Can you work these out from the model? Positions are in its coordinate system, mm. A direction names the side the tool comes from. Give positions to 0.01 mm unless a question says otherwise; leave off trailing zeros. Write each loop counter-clockwise with the first axis right and the second up, starting at its lowest first coordinate (ties: lowest second). Pieces come first, ordered by that corner, then holes. Notation, with made-up numbers: (49, 0.25) -> (90, 0.25) arc R23 ccw to (90, 37.25) -> close; hole circle Ø6 at (59, -33). An arc over 180 degrees is marked (long way). One line per item, written item: value.
from build123d import *

# Parameters (mm, degrees)
SKETCH1_W           = 40
SKETCH1_H           = 20
SKETCH1_R           = 4
BOSS_EXTRUDE1_DEPTH = 38
SKETCH1_3_R         = 4
BOSS_EXTRUDE2_DEPTH = 6
SKETCH2_R           = 6.5
BOSS_EXTRUDE3_DEPTH = 2
SKETCH3_W           = 7
SKETCH3_H           = 20
SKETCH3_R           = 2.25
BOSS_EXTRUDE4_DEPTH = 2.5


with BuildPart() as part:
    # Sketch1 → Boss-Extrude1 (new body)
    # profile 1 of 2: a face of its own
    with BuildSketch(Plane(origin=(0, 0, 0), x_dir=(1, 0, 0), z_dir=(0, 1, 0))):
        with Locations((-11, 0)):
            Rectangle(SKETCH1_W, SKETCH1_H)
        Circle(SKETCH1_R, mode=Mode.SUBTRACT)
    # profile 2 of 2: a face of its own
    with BuildSketch(Plane(origin=(0, 0, 0), x_dir=(1, 0, 0), z_dir=(0, 1, 0))):
        Circle(SKETCH1_R)
    extrude(amount=-BOSS_EXTRUDE1_DEPTH)

    # Sketch1_3 → Boss-Extrude2 (add)
    with BuildSketch(Plane(origin=(0, 0, 0), x_dir=(1, 0, 0), z_dir=(0, 1, 0))):
        with Locations(Location((0, 0, 0), (0, 0, 270))):
            Circle(SKETCH1_3_R)
    extrude(amount=BOSS_EXTRUDE2_DEPTH)

    # Sketch2 → Boss-Extrude3 (add)
    with BuildSketch(Plane(origin=(0, 0, 0), x_dir=(1, 0, 0), z_dir=(0, 1, 0))):
        with Locations(Location((0, 0, 0), (0, 0, 270))):
            Circle(SKETCH2_R)
    extrude(amount=BOSS_EXTRUDE3_DEPTH)


with BuildPart() as body_2:
    # Sketch3 → Boss-Extrude4 (new body)
    with BuildSketch(Plane(origin=(0, -8, 0), x_dir=(-1, 0, 0), z_dir=(0, -1, 0))):
        with Locations((-12.5, 0)):
            Rectangle(SKETCH3_W, SKETCH3_H)
        with Locations(Location((-13.5, 5, 0), (0, 0, 90))):
            Circle(SKETCH3_R, mode=Mode.SUBTRACT)
        with Locations(Location((-13.5, -5, 0), (0, 0, 90))):
            Circle(SKETCH3_R, mode=Mode.SUBTRACT)
    extrude(amount=BOSS_EXTRUDE4_DEPTH)


with BuildPart() as body_3:
    # Mirror1: mirrored copy
    add(body_2.part.mirror(Plane(origin=(-11, 0, 0), x_dir=(0, 0, 1), z_dir=(1, 0, 0))))

    # Combine1: union part, body 2
    add(part.part)
    add(body_2.part)


solid = body_3.part
1) For faces 1 (the face through (-35, -10.5, 0)), 2 (the face through (3, 2, 3)), 3 (the face through (-31, -4, 0)), 4 (the face through (9, -24, 0)), 5 (the face through (13, -8, 0)), which set-ups out of +Z, -Z, +X, -X, +Y, -Y let a thin tool reach every point of the face, with its end or its side?
Answer list:
face 1: +Z, -Z, -X, -Y
face 2: +Y
face 3: +Z, -Z, -X, +Y
face 4: +Z, -Z, +X, -Y
face 5: +Z, -Z, +X, +Y
2) If we section it at C-C (x = 0): Write out the boundary of the cut face in (y, z), and give its area (3 significant figures).
Answer list:
outline: (-38, -10) -> (0, -10) -> (0, -6.5) -> (2, -6.5) -> (2, -4) -> (6, -4) -> (6, 4) -> (2, 4) -> (2, 6.5) -> (0, 6.5) -> (0, 10) -> (-38, 10) -> close
area: 818 mm^2
3) I need wall thicknesses on L1, parallel to X at y = -8.95, z = -5; L2, parallel to Z at x = -35.5, y = -9.3; L3, parallel to Y at x = 5, z = -4.75. Which ranges of each line are inside material? Lowest first, please.
Answer list:
L1: x = -38 to -37.75, -33.25 to 11.25, 15.75 to 16
L2: z = -10 to -7.25, -2.75 to 2.75, 7.25 to 10
L3: y = -38 to 0
4) Will these pins go through, and if not, where does the flat tip stop? pin 1 (5.5 mm diameter, centred on x = 12.5, z = -4.5, fed in from -Y); pin 2 (2 mm diameter, centred on y = -13.5, z = 3.5, fed in from +X); pin 3 (10 mm diameter, centred on y = -31.5, z = 5, fed in from -X); pin 4 (6 mm diameter, centred on x = -1, z = -5, fed in from +Y).
Answer list:
pin 1: stops at y = -10.5
pin 2: stops at x = 9
pin 3: stops at x = -31
pin 4: stops at y = 6
5) If we section it at A-A (x = 13.5): Write out the boundary of the cut face in (y, z).
Answer list:
outline: (-10.5, -10) -> (-8, -10) -> (-8, -7.25) -> (-10.5, -7.25) -> close; (-10.5, -2.75) -> (-8, -2.75) -> (-8, 2.75) -> (-10.5, 2.75) -> close; (-10.5, 7.25) -> (-8, 7.25) -> (-8, 10) -> (-10.5, 10) -> close
6) If we section it at B-B (z = 5): Write out the boundary of the cut face in (x, y), and give its area (3 significant figures).
Answer list:
outline: (-38, -10.5) -> (-37.75, -10.5) -> (-37.75, -8) -> (-38, -8) -> close; (-33.25, -10.5) -> (-31, -10.5) -> (-31, -38) -> (9, -38) -> (9, -10.5) -> (11.25, -10.5) -> (11.25, -8) -> (9, -8) -> (9, 0) -> (4.15, 0) -> (4.15, 2) -> (-4.15, 2) -> (-4.15, 0) -> (-31, 0) -> (-31, -8) -> (-33.25, -8) -> close; (15.75, -10.5) -> (16, -10.5) -> (16, -8) -> (15.75, -8) -> close
area: 1,550 mm^2
7) If we section it at D-D (z = 0): Write out the boundary of the cut face in (x, y), and give its area (3 significant figures).
Answer list:
outline: (-38, -10.5) -> (-31, -10.5) -> (-31, -38) -> (9, -38) -> (9, -10.5) -> (16, -10.5) -> (16, -8) -> (9, -8) -> (9, 0) -> (6.5, 0) -> (6.5, 2) -> (4, 2) -> (4, 6) -> (-4, 6) -> (-4, 2) -> (-6.5, 2) -> (-6.5, 0) -> (-31, 0) -> (-31, -8) -> (-38, -8) -> close
area: 1,610 mm^2
